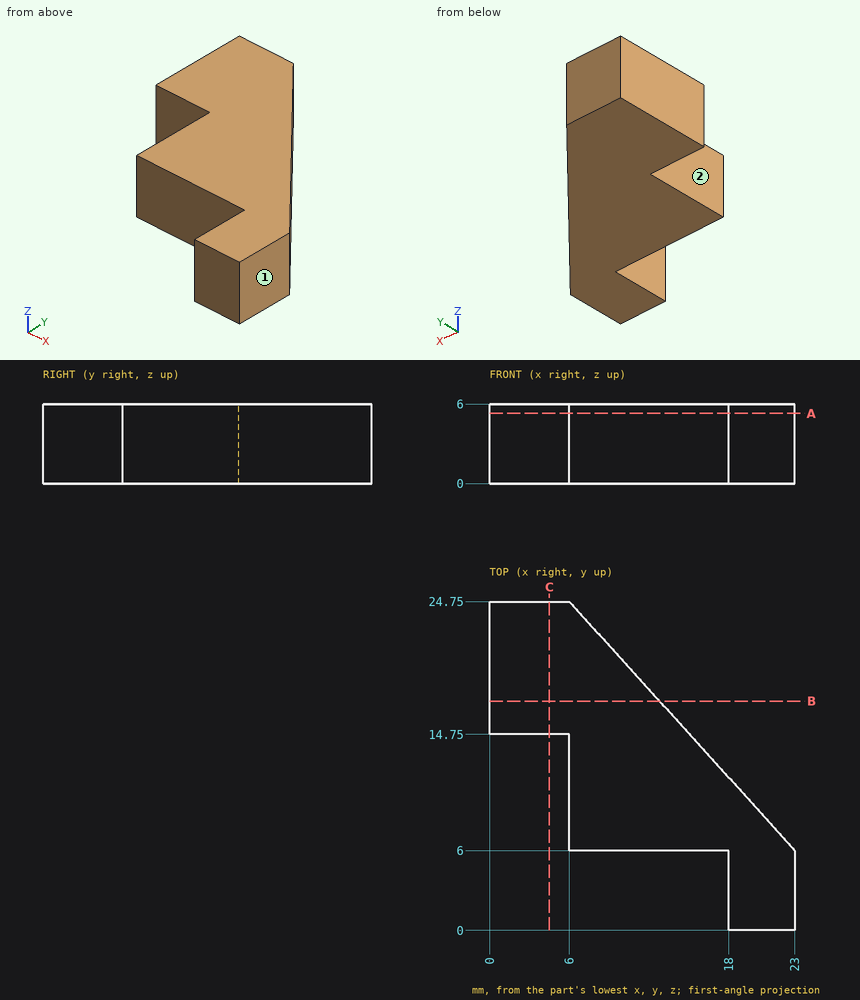
Could you check a few things on this drawing? It's one solid part, dimensions in mm from its lowest x, y, z. A direction names the side the tool comes from. Round coordinates to 2 decimals unless told otherwise and drop trailing zeros. Order: outer loops, then holes, each group sorted by start corner. A loop starts at its lowest first (then second) coordinate and runs counter-clockwise, first axis right, second up. Notation, with made-up numbers: (18.25, 42) -> (40.25, 42) arc R25 ccw to (40.25, 77) -> close; hole circle Ø5 at (-2.75, -29). An arc over 180 degrees is marked (long way). One line per question, with ' | ' between items.
Q1. If we section it at C-C on x = 4.5: Write out the boundary of the cut face in (y, z), plus the area to 3 significant figures.
Computed values:
outline: (14.75, 0) -> (24.75, 0) -> (24.75, 6) -> (14.75, 6) -> close | area: 60.0 mm²
Q2. If we section it at A-A on z = 5.3: Write out the boundary of the cut face in (x, y), plus the area to 3 significant figures.
Computed values:
outline: (0, 14.75) -> (6, 14.75) -> (6, 6) -> (18, 6) -> (18, 0) -> (23, 0) -> (23, 6) -> (6, 24.75) -> (0, 24.75) -> close | area: 249 mm²
Q3. I'm going to push flat-ended pins straight in: pin 1 (1 mm diameter, centred on x = 15.5, z = 5.5, fed in from -Y); pin 2 (3 mm diameter, centred on y = 3.5, z = 4, fed in from -X); pin 3 (1 mm diameter, centred on x = 20, z = 1.5, fed in from +Y). Where does each tip first touch, or does it pass through?
Computed values:
pin 1: y = 6 | pin 2: x = 18 | pin 3: y = 9.86
Q4. Which directions (+Z, -Z, +X, -X, +Y, -Y) give clear straight access to the entire face, cutting with the end or side of a thin tool? Please do the marked faces 1 and 2.
Computed values:
face 1: +Z, -Z, +X, +Y, -Y | face 2: +Z, -Z, -X, -Y
Q5. If we section it at B-B on y = 17.25: Write out the boundary of the cut face in (x, z), plus the area to 3 significant figures.
Computed values:
outline: (0, 0) -> (12.8, 0) -> (12.8, 6) -> (0, 6) -> close | area: 76.8 mm²
Q6. If I drill on line 1 (X direction, y = 4.75, z = 2.9); line 2 (Y direction, x = 1.25, z = 0.9); line 3 (Y direction, x = 19, z = 4.4), over which ranges is the centre line in solid material (lowest first)? Write a range as from..to.
Computed values:
line 1: 18..23 | line 2: 14.75..24.75 | line 3: 0..10.41
